Here's how the part is built. I have some questions about the finished solid (model axes, mm). Face numbers are marked on the shaded views. A direction names the side the tool comes from. Coordinates: 2 decimals unless noted, no trailing zeros. Loops run counter-clockwise (first coordinate to the right, second up) from the corner with the lowest first, then second, coordinate; pieces in that order, holes last. Notation, with made-up numbers: (-2.5, 35) -> (54.5, 35) arc R21 ccw to (54.5, 43) -> close; hole circle Ø11 at (78.25, -29.75). An arc over 180 degrees is marked (long way). Answer as a JSON object with one key per item and string values. Group by question number.
1) Which directions (+Z, -Z, +X, -X, +Y, -Y) give clear straight access to the entire face, cutting with the end or side of a thin tool? Please do the marked faces 1 and 2.
2) I want a section at B-B (z = -1.55). Write out the boundary of the cut face in (x, y).
3) If we mould it in two halves opening along Y, with no side actions, what happens to the marked faces 3, 4, 5 and 6? For each: +Y half, -Y half, draft (parallel to the pull), parting line (faces both ways), or undercut.
4) I need wall thicknesses on probe 1 along X at (y, z) = (1.25, -0.7); probe 2 along Y at (x, z) = (35, -1.1). Which ranges of each line are inside material? Lowest first, please. Write a range as [from, to].
5) I'm going to push a flat-ended pin straight in: pin 1 (2 mm diameter, centred on x = 34, y = 0, fed in from -Z) (3 decimals). Where does the tip first touch, or does it pass through?
6) I want a section at A-A (y = -1). Write out the boundary of the cut face in (x, z) (3 decimals), then the cut area to 3 significant figures.
```python
from build123d import *

# Parameters (mm, degrees)
SKETCH1_W           = 39.86221147
SKETCH1_H           = 6.35
SKETCH1_W_2         = 3.175
SKETCH1_H_2         = 3.175
BOSS_EXTRUDE1_DEPTH = 3.175


with BuildPart() as part:
    # Sketch1 → Boss-Extrude1 (new body)
    with BuildSketch(Plane.XY):
        with Locations((43.507685092, -0.004486266)):
            Rectangle(SKETCH1_W, SKETCH1_H)
        with Locations((54.362348302, -0.004486266)):
            Rectangle(SKETCH1_W_2, SKETCH1_H_2, mode=Mode.SUBTRACT)
        with Locations((35.358431187, -0.004486266)):
            Rectangle(SKETCH1_W_2, SKETCH1_H_2, mode=Mode.SUBTRACT)
    extrude(amount=-BOSS_EXTRUDE1_DEPTH)


solid = part.part
```
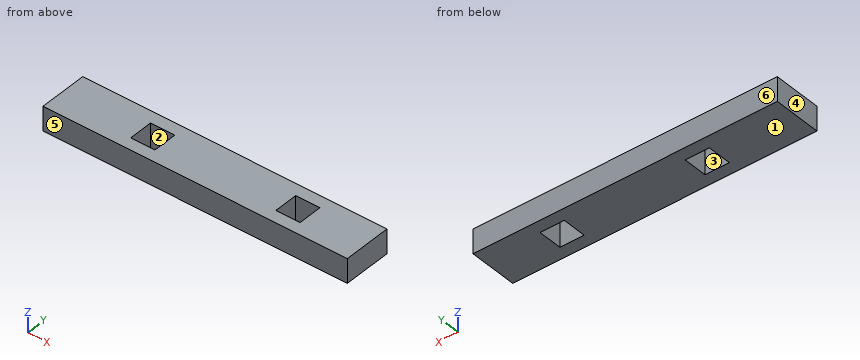
Determined:
{
 "1": {"face 1": "-Z, +X, -X, +Y, -Y", "face 2": "+Z, -Z"},
 "2": {"outline": "(23.58, -3.18) -> (63.44, -3.18) -> (63.44, 3.17) -> (23.58, 3.17) -> close; hole (33.77, -1.59) -> (36.95, -1.59) -> (36.95, 1.58) -> (33.77, 1.58) -> close; hole (52.77, -1.59) -> (55.95, -1.59) -> (55.95, 1.58) -> (52.77, 1.58) -> close"},
 "3": {"face 3": "undercut", "face 4": "draft", "face 5": "-Y half", "face 6": "+Y half"},
 "4": {"probe 1": "[23.58, 33.77], [36.95, 52.77], [55.95, 63.44]", "probe 2": "[-3.18, -1.59], [1.58, 3.17]"},
 "5": {"pin 1": "z = -3.175"},
 "6": {"outline": "(23.577, -3.175) -> (33.771, -3.175) -> (33.771, 0) -> (23.577, 0) -> close; (36.946, -3.175) -> (52.775, -3.175) -> (52.775, 0) -> (36.946, 0) -> close; (55.95, -3.175) -> (63.439, -3.175) -> (63.439, 0) -> (55.95, 0) -> close", "area": "106 mm^2"}
}
